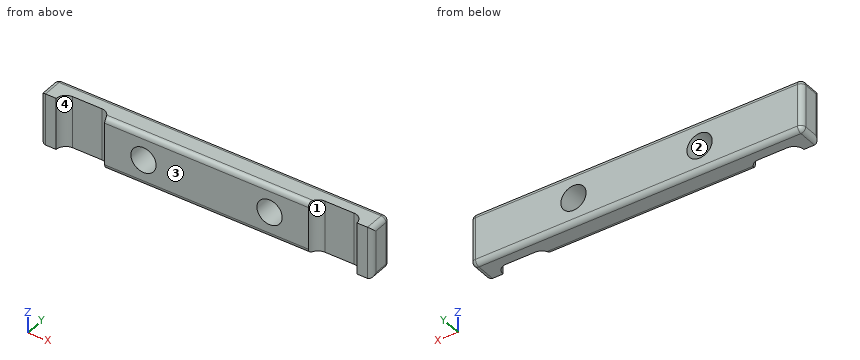
```python
from build123d import *

# Parameters (mm, degrees)
SKETCH1_W           = 68.4
SKETCH1_H           = 10.72
BOSS_EXTRUDE1_DEPTH = 5
CUT_EXTRUDE3_REACH  = 36.977
SKETCH6_R           = 2.6
CUT_EXTRUDE4_DEPTH  = 37.187821156
FILLET1_R           = 1
FILLET2_R           = 1
FILLET3_R           = 1


with BuildPart() as part:
    # Sketch1 → Boss-Extrude1 (new body)
    with BuildSketch(Plane(origin=(0, 0, 0), x_dir=(1, 0, 0), z_dir=(0, 1, 0))):
        Rectangle(SKETCH1_W, SKETCH1_H)
    extrude(amount=BOSS_EXTRUDE1_DEPTH)

    # Sketch6 → Cut-Extrude3 (cut, up to next)
    with BuildSketch(Plane(origin=(0, 0, 0), x_dir=(1, 0, 0), z_dir=(0, 1, 0)), mode=Mode.PRIVATE) as cut_extrude3_sk1:
        with Locations(Location((-13, 0, 0), (0, 0, 270))):
            Circle(SKETCH6_R)
    cut_extrude3_tool1 = extrude(cut_extrude3_sk1.sketch, amount=CUT_EXTRUDE3_REACH, mode=Mode.PRIVATE) & part.part
    cut_extrude3 = cut_extrude3_tool1.solids().sort_by_distance((-13, 0, 0))[0]
    add(cut_extrude3, mode=Mode.SUBTRACT)

    # Sketch9 → Cut-Extrude4 (cut, through all)
    with BuildSketch(Plane.XY.offset(5.36)):
        with BuildLine():
            Line((-23, 2), (-29, 2))
            ThreePointArc((-29, 2), (-30.414213562, 1.414213562), (-31, 0))
            Line((-31, 0), (-21, 0))
            ThreePointArc((-21, 0), (-21.585786438, 1.414213562), (-23, 2))
        make_face()
    cut_extrude4 = extrude(amount=-CUT_EXTRUDE4_DEPTH, mode=Mode.SUBTRACT)

    # Mirror4: Cut-Extrude4 across plane
    add(cut_extrude4.mirror(Plane(origin=(0, 0, 0), x_dir=(0, 0, 1), z_dir=(1, 0, 0))), mode=Mode.SUBTRACT)

    # Fillet1
    fillet1_edges = [part.edges().sort_by_distance(p)[0] for p in [
        (-34.2, 5, 0),
    ]]
    fillet(fillet1_edges, radius=FILLET1_R)

    # Fillet2
    fillet2_edges = [part.edges().sort_by_distance(p)[0] for p in [
        (34.2, 5, 0),
    ]]
    fillet(fillet2_edges, radius=FILLET2_R)

    # Mirror5: Cut-Extrude3 across plane
    add(cut_extrude3.mirror(Plane(origin=(0, 0, 0), x_dir=(0, 0, 1), z_dir=(1, 0, 0))), mode=Mode.SUBTRACT)

    # Fillet3
    fillet3_edges = [part.edges().sort_by_distance(p)[0] for p in [
        (-34.2, 2, 5.36),
        (-33.907106781, 4.707106781, 5.36),
        (34.2, 2, 5.36),
        (33.907106781, 4.707106781, 5.36),
        (34.2, 2, -5.36),
        (33.907106781, 4.707106781, -5.36),
        (-34.2, 2, -5.36),
        (-33.907106781, 4.707106781, -5.36),
        (34.2, 0, 0),
        (-34.2, 0, 0),
        (0, 5, 5.36),
        (0, 5, -5.36),
        (0, 0, 5.36),
        (0, 0, -5.36),
    ]]
    fillet(fillet3_edges, radius=FILLET3_R)


solid = part.part
```
Source: CAD feature listing. Evaluate the final solid. Frame: model axes, mm. Face numbers are marked on the shaded views. A direction names the side the tool comes from. Coordinates: 2 decimals unless noted, no trailing zeros. Loops run counter-clockwise (first coordinate to the right, second up) from the corner with the lowest first, then second, coordinate; pieces in that order, holes last. Notation, with made-up numbers: M 70,4.5 L 123,4.5 A19 ccw 123,15.5 Z; hole C 20.25,-21 d5. An arc over 180 degrees is marked long. Use a Markdown table: item, result. Add a question column.
Q1. Access query for the marked faces 1 and 2. Directions: +Z, -Z, +X, -X, +Y, -Y. A direction counts if a zero-diameter tool reaches every point of the face in a straight line with its end or side. Return the directions, or none.
Q2. Section query C-C, the plane z = 3.75. Return loops of the section in (x, y).
Q3. Section query D-D, the plane y = 2.85. Return loops of the section in (x, z), and give its area (3 significant figures).
Q4. Section query A-A, the plane x = 13. Return loops of the section in (y, z), and give its area (3 significant figures).
Q5. First-contact query: pin 1 (1.8 mm diameter, centred on x = 26.5, z = 1.5, fed in from -Y). Flat tip, straight axial feed; report the tip coordinate or a pass-through.
Q6. Draft query along X for the marked faces 3 and 4. Return one class per face: pulls with the +X half, pulls with the -X half, needs draft (parallel to the pull), parting line crosses it, or undercut.
Q7. Material intervals for L1, parallel to X at y = 2.6, z = 0; L2, parallel to Z at x = 13, y = 1.6; L3, parallel to X at y = 1, z = -0.5, sorted ascending.
Q8. Section query B-B, the plane z = 0. Return loops of the section in (x, y).
Result:
| question | item | result |
|---|---|---|
| 1 | face 1 | +Z, -Z, -Y |
| 1 | face 2 | +Y, -Y |
| 2 | outline | M -34.2,1 A1 ccw -33.2,0 L -31,0 A2 cw -29,2 L -23,2 A2 cw -21,0 L 21,0 A2 cw 23,2 L 29,2 A2 cw 31,0 L 33.2,0 A1 ccw 34.2,1 L 34.2,4 A1 ccw 33.2,5 L -33.2,5 A1 ccw -34.2,4 Z |
| 3 | outline | M -34.2,-4.36 A1 ccw -33.2,-5.36 L 33.2,-5.36 A1 ccw 34.2,-4.36 L 34.2,4.36 A1 ccw 33.2,5.36 L -33.2,5.36 A1 ccw -34.2,4.36 Z; hole C -13,0 d5.2; hole C 13,0 d5.2 |
| 3 | area | 690 mm2 |
| 4 | outline | M 0,-4.36 A1 ccw 1,-5.36 L 4,-5.36 A1 ccw 5,-4.36 L 5,-2.6 L 0,-2.6 Z; M 0,2.6 L 5,2.6 L 5,4.36 A1 ccw 4,5.36 L 1,5.36 A1 ccw 0,4.36 Z |
| 4 | area | 26.7 mm2 |
| 5 | pin 1 | stops at y = 2 |
| 6 | face 3 | needs draft |
| 6 | face 4 | undercut |
| 7 | L1 | x = -34.2 to -15.6, -10.4 to 10.4, 15.6 to 34.2 |
| 7 | L2 | z = -5.36 to -2.6, 2.6 to 5.36 |
| 7 | L3 | x = -34.2 to -30.73, -21.27 to -15.55, -10.45 to 10.45, 15.55 to 21.27, 30.73 to 34.2 |
| 8 | outline | M -34.2,1 A1 ccw -33.2,0 L -31,0 A2 cw -29,2 L -23,2 A2 cw -21,0 L -15.6,0 L -15.6,5 L -33.2,5 A1 ccw -34.2,4 Z; M -10.4,0 L 10.4,0 L 10.4,5 L -10.4,5 Z; M 15.6,0 L 21,0 A2 cw 23,2 L 29,2 A2 cw 31,0 L 33.2,0 A1 ccw 34.2,1 L 34.2,4 A1 ccw 33.2,5 L 15.6,5 Z |
